Can you work these out from the model? Positions are in its coordinate system, mm. Face numbers are marked on the shaded views. A direction names the side the tool comes from. Round coordinates to 2 decimals unless told otherwise and drop trailing zeros. Loops run counter-clockwise (first coordinate to the right, second up) from the corner with the lowest first, then second, coordinate; pieces in that order, holes last.
from build123d import *

# Parameters (mm, degrees)
SKETCH_W        = 59
SKETCH_H        = 10
PAD_DEPTH       = 3
POCKET_DEPTH    = 10.001
POCKET001_DEPTH = 3.001


with BuildPart() as part:
    # Sketch → Pad (new body)
    with BuildSketch(Plane.XY):
        with Locations((29.5, 5)):
            Rectangle(SKETCH_W, SKETCH_H)
    extrude(amount=PAD_DEPTH)

    # Sketch001 (on Face3 of Pad) → Pocket (cut, through all)
    with BuildSketch(Plane.XZ):
        Polygon((0, 0), (3, 3), (0, 3), align=None)
    extrude(amount=-POCKET_DEPTH, mode=Mode.SUBTRACT)

    # Sketch002 (on Face4 of Pocket) → Pocket001 (cut, through all)
    with BuildSketch(Plane.XY.offset(3)):
        with BuildLine():
            ThreePointArc((10, 7.5), (7.5, 5), (10, 2.5))
            Line((10, 2.5), (15, 2.5))
            ThreePointArc((15, 2.5), (17.5, 5), (15, 7.5))
            Line((10, 7.5), (15, 7.5))
        make_face()
        with BuildLine():
            ThreePointArc((46, 2.5), (48.5, 5), (46, 7.5))
            Line((46, 7.5), (41, 7.5))
            ThreePointArc((41, 7.5), (38.5, 5), (41, 2.5))
            Line((46, 2.5), (41, 2.5))
        make_face()
    extrude(amount=-POCKET001_DEPTH, mode=Mode.SUBTRACT)


solid = part.part
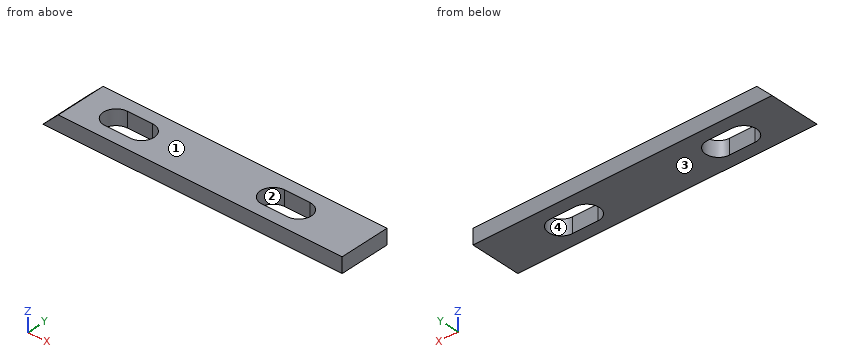
(1) If we section it at A-A, the plane x = 42: List the corners of the cut face in (y, z) for me, then the cut area to 3 significant figures.
Worked answers:
outline: (0, 0) - (2.5, 0) - (2.5, 3) - (0, 3) - close; (7.5, 0) - (10, 0) - (10, 3) - (7.5, 3) - close
area: 15.0 mm2
(2) If we mould it in two halves opening along X, with no side actions, what happens to the marked faces 1 and 2? For each: released by +X, released by -X, zero draft, split by the parting line, or undercut.
Worked answers:
face 1: zero draft
face 2: undercut
(3) If I drill on line 1 (X direction, y = 2.75, z = 1.45); line 2 (X direction, y = 3.5, z = 0.9); line 3 (Y direction, x = 42, z = 0.7), over which ranges is the centre line in solid material (lowest first)?
Worked answers:
line 1: x = 1.45 to 8.91, 16.09 to 39.91, 47.09 to 59
line 2: x = 0.9 to 8, 17 to 39, 48 to 59
line 3: y = 0 to 2.5, 7.5 to 10
(4) Will this pin go through, and if not, where does the flat tip stop? P1, Ø1, axis at x = 53, y = 5.5, coming from the -Z side.
Worked answers:
P1: stops at z = 0
(5) If we section it at B-B, the plane z = 1.2: List the corners of the cut face in (x, y) for me, then the cut area to 3 significant figures.
Worked answers:
outline: (1.2, 0) - (59, 0) - (59, 10) - (1.2, 10) - close; hole (10, 2.5) - (15, 2.5) arc R2.5 ccw to (15, 7.5) - (10, 7.5) arc R2.5 ccw to start; hole (41, 2.5) - (46, 2.5) arc R2.5 ccw to (46, 7.5) - (41, 7.5) arc R2.5 ccw to start
area: 489 mm2
(6) If we section it at D-D, the plane x = 15.5: List the corners of the cut face in (y, z) for me, then the cut area to 3 significant figures.
Worked answers:
outline: (0, 0) - (2.55, 0) - (2.55, 3) - (0, 3) - close; (7.45, 0) - (10, 0) - (10, 3) - (7.45, 3) - close
area: 15.3 mm2
(7) If we section it at C-C, the plane y = 5: List the corners of the cut face in (x, z) for me.
Worked answers:
outline: (0, 0) - (7.5, 0) - (7.5, 3) - (3, 3) - close; (17.5, 0) - (38.5, 0) - (38.5, 3) - (17.5, 3) - close; (48.5, 0) - (59, 0) - (59, 3) - (48.5, 3) - close
(8) For the marked faces 3 and 4, which set-ups out of +Z, -Z, +X, -X, +Y, -Y let a thin tool reach every point of the face, with its end or its side?
Worked answers:
face 3: -Z, +X, -X, +Y, -Y
face 4: +Z, -Z
